The listing builds one solid part. Answer for the finished solid, in the listing's coordinates (mm). Give positions to 0.01 mm unless a question says otherwise; leave off trailing zeros. Write each loop counter-clockwise with the first axis right and the second up, starting at its lowest first coordinate (ties: lowest second). Pieces come first, ordered by that corner, then holes. Notation, with made-up numbers: (34.25, 13) - (77.25, 13) arc R7 ccw to (77.25, 20) - close; hole circle Ø5 at (-10, 60.25). An arc over 180 degrees is marked (long way). Use a Markdown table: item, result. Add a question column.
from build123d import *

# Parameters (mm, degrees)
F0_W     = 130.451084
F0_H     = 101.461962
F1_DEPTH = 63.5
F2_R     = 27.0412
F3_DEPTH = 50.8
F4_R     = 18.876355
F5_DEPTH = 179.578


with BuildPart() as f1:
    # F0 (on Front) → F1 (new body)
    with BuildSketch(Plane.XZ):
        Rectangle(F0_W, F0_H)
    extrude(amount=F1_DEPTH)

    # F2 (on face) → F3 (join)
    with BuildSketch(Plane.XZ.offset(63.5)):
        Circle(F2_R)
    extrude(amount=F3_DEPTH)

    # F4 (on face) → F5 (cut)
    with BuildSketch(Plane.XZ.offset(114.3)):
        Circle(F4_R)
    extrude(amount=-F5_DEPTH, mode=Mode.SUBTRACT)


solid = f1.part
1. The part is cut by section A-A (z = 0). Give the vertices of the cut face in (x, y), and give its area (3 significant figures).
2. Given P1, Ø1, axis at x = -28, z = -34.5, coming from the -Y side; P2, Ø2, axis at x = -7, y = -83.5, coming from the -Z side, each flat-ended and moving along its own axis, determine where each tip first touches the part or whether it passes through.
3. The part is cut by section C-C (y = -16). Give the vertices of the cut face in (x, z).
4. For a pull along X with two mould halves and no side action, classify faces 1 (the cylindrical face through (-14.98, -57.95, -11.486)), 2 (the cylindrical face through (-5.86, -88.54, -26.4)), 3 (the flat face through (5.6, -114.3, 18.4)) as released by +X, released by -X, zero draft, split by the parting line, or undercut.
5. The part is cut by section B-B (x = 0). Give the vertices of the cut face in (y, z).
6. The part is cut by section D-D (z = 41.5). Give the vertices of the cut face in (x, y).
7. Consider L1, parallel to X at y = -85.5, z = -0.5; L2, parallel to Z at x = 0, y = -67; L3, parallel to Y at x = 24.5, z = -19. Determine where each line is inside the solid, lowest interval first. Write a range as [from, to].
Check values:
| question | item | result |
|---|---|---|
| 1 | outline | (-65.23, -63.5) - (-27.04, -63.5) - (-27.04, -114.3) - (-18.88, -114.3) - (-18.88, 0) - (-65.23, 0) - close; (18.88, -114.3) - (27.04, -114.3) - (27.04, -63.5) - (65.23, -63.5) - (65.23, 0) - (18.88, 0) - close |
| 1 | area | 6,720 mm2 |
| 2 | P1 | stops at y = -63.5 |
| 2 | P2 | stops at z = -26.37 |
| 3 | outline | (-65.23, -50.73) - (65.23, -50.73) - (65.23, 50.73) - (-65.23, 50.73) - close; hole circle Ø37.75 at (0, 0) |
| 4 | face 1 | undercut |
| 4 | face 2 | split by the parting line |
| 4 | face 3 | zero draft |
| 5 | outline | (-114.3, -27.04) - (-63.5, -27.04) - (-63.5, -50.73) - (0, -50.73) - (0, -18.88) - (-114.3, -18.88) - close; (-114.3, 18.88) - (0, 18.88) - (0, 50.73) - (-63.5, 50.73) - (-63.5, 27.04) - (-114.3, 27.04) - close |
| 6 | outline | (-65.23, -63.5) - (65.23, -63.5) - (65.23, 0) - (-65.23, 0) - close |
| 7 | L1 | x = [-27.04, -18.87], [18.87, 27.04] |
| 7 | L2 | z = [-27.04, -18.88], [18.88, 27.04] |
| 7 | L3 | y = [-63.5, 0] |
